```python
from build123d import *

# Parameters (mm, degrees)
SKETCH1_W           = 600
SKETCH1_H           = 200
SKETCH1_R           = 2.25
SKETCH1_W_2         = 50
SKETCH1_H_2         = 100
SKETCH1_W_3         = 20
SKETCH1_H_3         = 5
SKETCH1_W_4         = 72
SKETCH1_H_4         = 25
BOSS_EXTRUDE1_DEPTH = 4


with BuildPart() as part:
    # Sketch1 → Boss-Extrude1 (new body)
    with BuildSketch(Plane.XY):
        with Locations((300, 100)):
            Rectangle(SKETCH1_W, SKETCH1_H)
        with Locations((220, 106.30966113)):
            Circle(SKETCH1_R, mode=Mode.SUBTRACT)
        with Locations((220, 6.19033887)):
            Circle(SKETCH1_R, mode=Mode.SUBTRACT)
        with Locations((125, 52.5)):
            Rectangle(SKETCH1_W_2, SKETCH1_H_2, mode=Mode.SUBTRACT)
        with Locations((50, 37.5)):
            Rectangle(SKETCH1_W_3, SKETCH1_H_3, mode=Mode.SUBTRACT)
        with Locations((50, 92.5)):
            Rectangle(SKETCH1_W_4, SKETCH1_H_4, mode=Mode.SUBTRACT)
        with BuildLine():
            ThreePointArc((234.957275327, 83.37125), (238, 72.2), (241.042724673, 83.37125))
            ThreePointArc((241.042724673, 83.37125), (240.684092439, 83.732653501), (240.549888987, 84.223794014))
            ThreePointArc((240.549888987, 84.223794014), (238, 86.75), (235.450111013, 84.223794014))
            ThreePointArc((235.450111013, 84.223794014), (235.315907561, 83.732653501), (234.957275327, 83.37125))
        make_face(mode=Mode.SUBTRACT)
    extrude(amount=BOSS_EXTRUDE1_DEPTH)


solid = part.part
```
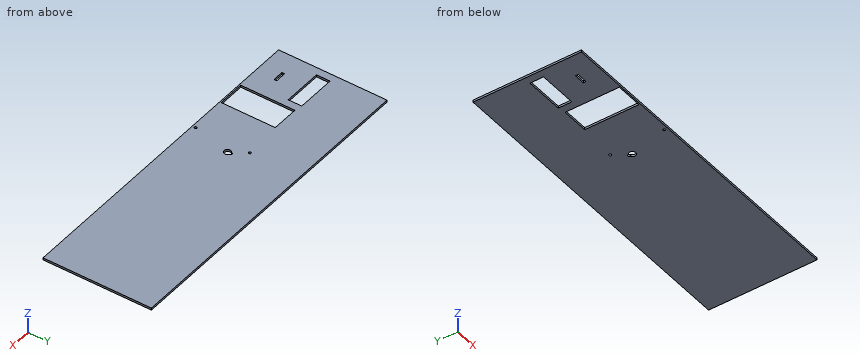
Input: part model. Units: mm. Frame: model coordinates. Give positions to 0.01 mm unless a question says otherwise; leave off trailing zeros. Order: outer loops, then holes, each group sorted by start corner. A loop starts at its lowest first (then second) coordinate and runs counter-clockwise, first axis right, second up.
1. Cut plane B-B (y = 52.5). Return loops of the section in (x, z), and give its area (3 significant figures).
Computed:
outline: (0, 0) - (100, 0) - (100, 4) - (0, 4) - close; (150, 0) - (600, 0) - (600, 4) - (150, 4) - close
area: 2,200 mm2
2. Cut plane C-C (z = 0.8). Return loops of the section in (x, y).
Computed:
outline: (0, 0) - (600, 0) - (600, 200) - (0, 200) - close; hole (14, 80) - (86, 80) - (86, 105) - (14, 105) - close; hole (40, 35) - (60, 35) - (60, 40) - (40, 40) - close; hole (100, 2.5) - (150, 2.5) - (150, 102.5) - (100, 102.5) - close; hole circle Ø4.5 at (220, 6.19); hole circle Ø4.5 at (220, 106.31); hole (234.96, 83.37) arc R6 ccw (long way) to (241.04, 83.37) arc R1 cw to (240.55, 84.22) arc R2.55 ccw to (235.45, 84.22) arc R1 cw to start
3. Cut plane A-A (x = 121). Return loops of the section in (y, z).
Computed:
outline: (0, 0) - (2.5, 0) - (2.5, 4) - (0, 4) - close; (102.5, 0) - (200, 0) - (200, 4) - (102.5, 4) - close
4. Pin query (flat end, axial travel): pin 1 Ø2 at (x, y) = (536.5, 103) entering from -Z. Return the tip coordinate at first contact, or that it passes through.
Computed:
pin 1: stops at z = 0
5. Line query: probe 1 along X at (y, z) = (102, 3.65); probe 2 along X at (y, z) = (78.2, 2.65); probe 3 along Y at (x, z) = (220, 2.3). Output: solid intervals per line, ascending.
Computed:
probe 1: x = 0 to 14, 86 to 100, 150 to 600
probe 2: x = 0 to 100, 150 to 232, 244 to 600
probe 3: y = 0 to 3.94, 8.44 to 104.06, 108.56 to 200
